The listing builds one solid part. Answer for the finished solid, in the listing's coordinates (mm). A direction names the side the tool comes from. Round coordinates to 2 decimals unless told otherwise and drop trailing zeros. Write each loop counter-clockwise with the first axis right and the second up, starting at its lowest first coordinate (ties: lowest second). Pieces come first, ordered by that corner, then holes. Notation, with made-up numbers: (78, -34) - (86, -34) arc R23 cw to (86, -19) - close; hole circle Ø5 at (70.5, 25). An arc over 180 degrees is marked (long way). Return JSON: item names as keys, results as strings. Group by question number.
(1) Section A-A, the plane x = 0 is taken. Write down the section's boundary in (y, z), then the cut area to 3 significant figures.
(2) Each of these flat-tipped pins is pushed along its axis until it touches: pin 1 (12 mm diameter, centred on y = 9.5, z = 132.5, fed in from -X); pin 2 (0.9 mm diameter, centred on x = -15.5, y = 15, fed in from +Z); pin 3 (6 mm diameter, centred on y = 2.5, z = -7.5, fed in from -X). Where does it stop, or does it pass through?
(3) Determine the mould class of faces 1 (the flat face through (-19.2, -19.1, -24.4)), 2 (the cylindrical face through (14, 15.43, 4.44)), 3 (the cylindrical face through (14, -15.57, 4.44)), 4 (the flat face through (18.822, 18.771, -9.86)) for opening direction X: +X half, -X half, draft (parallel to the pull), parting line (faces both ways), or undercut.
(4) Section D-D, the plane z = 73.5 is taken. Write down the section's boundary in (x, y), then the cut area to 3 significant figures.
(5) Section C-C, the plane y = 8 is taken. Write down the section's boundary in (x, z), then the cut area to 3 significant figures.
(6) Which of the six approach directions +Z, -Z, +X, -X, +Y, -Y give full straight-line access (tool end or side, diameter ignored) to faces 5 (the flat face through (0, -20.65, -10)), 6 (the flat face through (18.771, -18.822, -9.86)), 7 (the flat face through (-18.822, -18.771, -9.86)), 8 (the flat face through (-15, -15, 0))?
(7) Find the intervals of material crossed by line 1 along Y through (x, z) = (15.5, 7.25); line 2 along X through (y, z) = (15, 3), in increasing order. Write a range as [from, to].
(8) Section B-B, the plane z = -7.5 is taken. Write down the section's boundary in (x, y), then the cut area to 3 significant figures.
Autodesk Inventor part; units mm, degrees
ref_plane "YZ Plane" through (0, 0, 0) normal (1, 0, 0) x (0, 1, 0)
ref_plane "XZ Plane" through (0, 0, 0) normal (0, 1, 0) x (-1, 0, 0)
ref_plane "XY Plane" through (0, 0, 0) normal (0, 0, 1) x (1, 0, 0)
sketch "Sketch1" plane through (0, 0, 0) normal (0, 0, 1) x (1, 0, 0)
  line L0 (-21.15, -21.15) -> (21.15, -21.15)
  line L1 (21.15, -21.15) -> (21.15, 21.15)
  line L2 (21.15, 21.15) -> (-21.15, 21.15)
  line L3 (-21.15, 21.15) -> (-21.15, -21.15)
  line L4 (-21.15, -21.15) -> (21.15, 21.15) construction
  line L5 (21.15, -21.15) -> (-21.15, 21.15) construction
  line L6 (-15.5, -15.5) -> (15.5, -15.5) construction
  line L7 (15.5, -15.5) -> (15.5, 15.5) construction
  line L8 (15.5, 15.5) -> (-15.5, 15.5) construction
  line L9 (-15.5, 15.5) -> (-15.5, -15.5) construction
  line L10 (-15.5, -15.5) -> (15.5, 15.5) construction
  line L11 (15.5, -15.5) -> (-15.5, 15.5) construction
  circle A0 centre (-15.5, 15.5) radius 1.5
  circle A1 centre (15.5, 15.5) radius 1.5
  circle A2 centre (15.5, -15.5) radius 1.5
  circle A3 centre (-15.5, -15.5) radius 1.5
  point P0 (0, 0)
  dimension "d0" = 42.3
  dimension "d1" = 31
  dimension "d2" = 3
extrude "Extrusion1" add sketch "Sketch1" along normal blind 9
chamfer "Chamfer1" distance 4 angle 45 4 edges at (21.15, 21.15, 4.5) (21.15, -21.15, 4.5) (-21.15, 21.15, 4.5) (-21.15, -21.15, 4.5)
sketch "Sketch3" plane through (0, 0, 0) normal (0, 0, -1) x (-1, 0, 0)
  circle A0 centre (15.5, 15.5) radius 1.5
  line L0 (21.15, 17.15) -> (21.15, -17.15)
  line L1 (17.15, 21.15) -> (21.15, 17.15)
  line L2 (-17.15, 21.15) -> (17.15, 21.15)
  line L3 (-21.15, 17.15) -> (-17.15, 21.15)
  line L4 (-21.15, -17.15) -> (-21.15, 17.15)
  circle A1 centre (15.5, -15.5) radius 1.5
  circle A2 centre (-15.5, -15.5) radius 1.5
  circle A3 centre (-15.5, 15.5) radius 1.5
  circle A4 centre (15.5, 15.5) radius 1.5
  line L5 (21.15, -17.15) -> (17.15, -21.15)
  line L6 (21.15, 17.15) -> (21.15, -17.15)
  line L7 (17.15, 21.15) -> (21.15, 17.15)
  line L8 (-17.15, 21.15) -> (17.15, 21.15)
  line L9 (-21.15, 17.15) -> (-17.15, 21.15)
  line L10 (-21.15, -17.15) -> (-21.15, 17.15)
  line L11 (-17.15, -21.15) -> (-21.15, -17.15)
  line L12 (17.15, -21.15) -> (-17.15, -21.15)
  line L13 (-20.65, 16.9429) -> (-16.9429, 20.65)
  line L14 (-16.9429, 20.65) -> (16.9429, 20.65)
  line L15 (16.9429, 20.65) -> (20.65, 16.9429)
  line L16 (20.65, 16.9429) -> (20.65, -16.9429)
  line L17 (20.65, -16.9429) -> (16.9429, -20.65)
  line L18 (16.9429, -20.65) -> (-16.9429, -20.65)
  line L19 (-16.9429, -20.65) -> (-20.65, -16.9429)
  line L20 (-20.65, -16.9429) -> (-20.65, 16.9429)
  point P0 (0, 0)
  dimension "d8" = 0.5
  dimension "d10" = 0.5
  dimension "d11" = 0.5
  dimension "d12" = 0.5
extrude "Extrusion2" add sketch "Sketch3" along normal blind 20 contours A0 | A1 | A2 | A3 | L13 L14 L15 L16 L17 L18 L19 L20
sketch "Sketch4" plane through (0, 0, -20) normal (0, 0, -1) x (-1, 0, 0)
  line L0 (-21.15, 17.15) -> (-17.15, 21.15)
  line L1 (-17.15, 21.15) -> (17.15, 21.15)
  line L2 (17.15, 21.15) -> (21.15, 17.15)
  line L3 (21.15, 17.15) -> (21.15, -17.15)
  line L4 (21.15, -17.15) -> (17.15, -21.15)
  line L5 (17.15, -21.15) -> (-17.15, -21.15)
  line L6 (-17.15, -21.15) -> (-21.15, -17.15)
  line L7 (-21.15, -17.15) -> (-21.15, 17.15)
  point P0 (0, 0)
extrude "Extrusion3" add sketch "Sketch4" along normal blind 9
sketch "Sketch5" plane through (0, 0, 9) normal (0, 0, 1) x (1, 0, 0)
  circle A0 centre (0, 0) radius 11
  dimension "d17" = 22
extrude "Extrusion4" add sketch "Sketch5" along normal blind 1
sketch "Sketch6" plane through (0, 0, 10) normal (0, 0, 1) x (1, 0, 0)
  circle A0 centre (0, 0) radius 11
  circle A1 centre (0, 0) radius 4
  dimension "d20" = 8
extrude "Extrusion5" add sketch "Sketch6" along normal blind 150 contours A1
equation "\"d10\" = d8"
equation "\"d11\" = d8"
equation "\"d12\" = d8"
properties part number "StepperDrive"
Working result:
{
 "1": {"outline": "(-21.15, -29) - (21.15, -29) - (21.15, -20) - (20.65, -20) - (20.65, 0) - (21.15, 0) - (21.15, 9) - (11, 9) - (11, 10) - (4, 10) - (4, 160) - (-4, 160) - (-4, 10) - (-11, 10) - (-11, 9) - (-21.15, 9) - (-21.15, 0) - (-20.65, 0) - (-20.65, -20) - (-21.15, -20) - close", "area": "2,810 mm^2"},
 "2": {"pin 1": "stops at x = -1.94", "pin 2": "stops at z = 0", "pin 3": "stops at x = -20.65"},
 "3": {"face 1": "-X half", "face 2": "undercut", "face 3": "undercut", "face 4": "+X half"},
 "4": {"outline": "circle Ø8 at (0, 0)", "area": "50.3 mm^2"},
 "5": {"outline": "(-21.15, -29) - (21.15, -29) - (21.15, -20) - (20.65, -20) - (20.65, 0) - (21.15, 0) - (21.15, 9) - (7.55, 9) - (7.55, 10) - (-7.55, 10) - (-7.55, 9) - (-21.15, 9) - (-21.15, 0) - (-20.65, 0) - (-20.65, -20) - (-21.15, -20) - close", "area": "1,600 mm^2"},
 "6": {"face 5": "+X, -X, -Y", "face 6": "+X, -Y", "face 7": "-X, -Y", "face 8": "+Z"},
 "7": {"line 1": "y = [-21.15, -17], [-14, 14], [17, 21.15]", "line 2": "x = [-21.15, -16.91], [-14.09, 14.09], [16.91, 21.15]"},
 "8": {"outline": "(-20.65, -16.94) - (-16.94, -20.65) - (16.94, -20.65) - (20.65, -16.94) - (20.65, 16.94) - (16.94, 20.65) - (-16.94, 20.65) - (-20.65, 16.94) - close", "area": "1,680 mm^2"}
}
